Drawing for the job (mm, zero at the part's lowest x, y, z). A direction names the side the tool comes from. Give positions to 0.01 mm unless a question says otherwise; leave off trailing zeros. Order: outer loops, then holes, each group sorted by start corner. A loop starts at its lowest first (then second) coordinate and runs counter-clockwise, first axis right, second up. Notation, with made-up numbers: (79.5, -5.75) -> (134.5, -5.75) arc R20 ccw to (134.5, 13.25) -> close; hole circle Ø9 at (79, -1). An arc over 180 degrees is marked (long way). Use one line per item in the form item = value. Start each with the question number.
1) Probe line 1 (X direction, y = 77, z = 4) (1 decimal); line 2 (X direction, y = 41.5, z = 1) (1 decimal); line 3 (Y direction, x = 60, z = 6) (1 decimal). List the from-to ranges inside material, lowest first.
2) Cut at D-D, the plane y = 65.5. Give the cut face in (x, z) (1 decimal), and give its area (3 significant figures).
3) Drop flat-ended pins along their axis: P1, Ø2, axis at y = 51, z = 3, coming from the -X side; P2, Ø1, axis at y = 48.5, z = 3, coming from the +X side; P3, Ø2, axis at x = 44, z = 4.5, coming from the -Y side. Give the stop position or say it passes through.
4) Cut at C-C, the plane y = 37. Give the cut face in (x, z).
5) Tool access for the marked faces 1, 2, 3 and 4: list every direction of +Z, -Z, +X, -X, +Y, -Y with a clear straight run to the whole face (end or side of a thin tool).
6) Cut at A-A, the plane x = 60.5. Give the cut face in (y, z).
7) Mould opens along X. For the marked faces 5, 6 and 7 say: pulls with the +X half, pulls with the -X half, needs draft (parallel to the pull), parting line crosses it, or undercut.
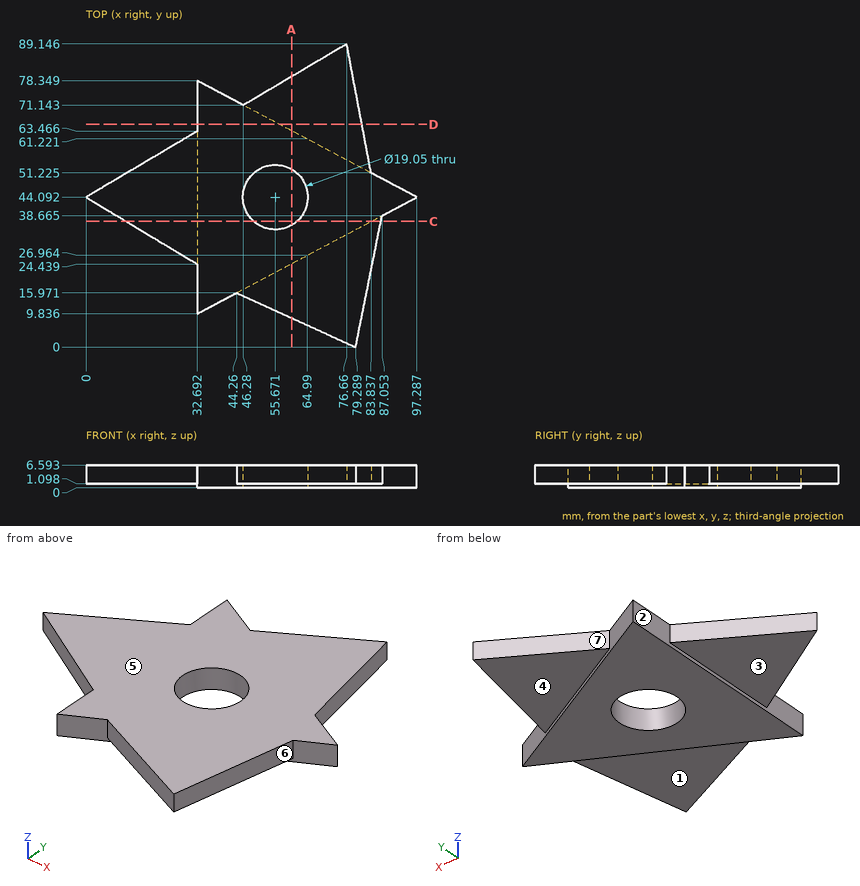
Result:
q1.line_1 = 32.7 to 35.2, 56.2 to 79
q1.line_2 = 32.7 to 46.5, 64.8 to 92.4
q1.line_3 = 8.8 to 35.6, 52.6 to 79.3
q2.outline = (32.7, 0) -> (56.9, 0) -> (56.9, 1.1) -> (81.1, 1.1) -> (81.1, 6.6) -> (32.7, 6.6) -> close
q2.area = 293 mm²
q3.P1 = 9.97
q3.P2 = 89.92
q3.P3 = 15.3
q4.outline = (11.8, 1.1) -> (32.69, 1.1) -> (32.69, 0) -> (49.31, 0) -> (49.31, 6.59) -> (11.8, 6.59) -> close; (62.03, 0) -> (83.91, 0) -> (83.91, 1.1) -> (86.72, 1.1) -> (86.72, 6.59) -> (62.03, 6.59) -> close
q5.face_1 = -Z, +X, -Y
q5.face_2 = -Z, -X
q5.face_3 = -Z, -X, +Y, -Y
q5.face_4 = -Z, +X, +Y
q6.outline = (8.57, 1.1) -> (24.58, 1.1) -> (24.58, 0) -> (35.88, 0) -> (35.88, 6.59) -> (8.57, 6.59) -> close; (52.3, 0) -> (63.6, 0) -> (63.6, 1.1) -> (79.57, 1.1) -> (79.57, 6.59) -> (52.3, 6.59) -> close
q7.face_5 = needs draft
q7.face_6 = pulls with the +X half
q7.face_7 = undercut
